Input: part model. Units: mm. Frame: model coordinates. A direction names the side the tool comes from. Coordinates: 2 decimals unless noted, no trailing zeros. Order: outer loops, then holes, each group sorted by start corner. A loop starts at its lowest first (then second) coordinate and runs counter-clockwise, first axis right, second up. Notation, with made-up numbers: M 61,-9.5 L 107,-9.5 A26 ccw 107,12.5 Z; hole C -19.5,46.25 d8. An arc over 180 degrees is marked long. Answer in a Markdown table with one row per item.
Autodesk Inventor part; units mm, degrees
ref_plane "Start plane" through (0, 0, -55) normal (0, 0, 1) x (1, 0, 0)
ref_plane "End plane" through (0, 0, 1555) normal (0, 0, 1) x (1, 0, 0)
ref_plane "Work Plane4" through (55, 0, 1555) normal (-0.7071, 0, 0.7071) x (0.7071, 0, 0.7071)
ref_plane "Start plane" through (0, 0, -55) normal (0, 0, 1) x (1, 0, 0)
ref_plane "End plane" through (0, 0, 1555) normal (0, 0, 1) x (1, 0, 0)
sketch "Sketch2" plane through (0, 0, 0) normal (0, 0, 1) x (1, 0, 0)
  line L0 (-55, 100.8) -> (-14.95, 100.8)
  line L1 (-55, 110) -> (-55, 100.8)
  line L2 (55, 110) -> (-55, 110)
  line L3 (55, 100.8) -> (55, 110)
  line L4 (14.95, 100.8) -> (55, 100.8)
  line L5 (2.95, -88.8) -> (2.95, 88.8)
  line L6 (55, -100.8) -> (14.95, -100.8)
  line L7 (55, -110) -> (55, -100.8)
  line L8 (-55, -100.8) -> (-55, -110)
  line L9 (-14.95, -100.8) -> (-55, -100.8)
  line L10 (-2.95, 88.8) -> (-2.95, -88.8)
  line L11 (0, -154) -> (0, 154) construction
  line L12 (-2.95, -100.8) -> (2.95, -100.8) construction
  arc A0 (-14.95, -100.8) -> (-2.95, -88.8) centre (-14.95, -88.8) ccw
  arc A1 (-2.95, 88.8) -> (-14.95, 100.8) centre (-14.95, 88.8) ccw
  arc A2 (14.95, 100.8) -> (2.95, 88.8) centre (14.95, 88.8) ccw
  arc A3 (2.95, -88.8) -> (14.95, -100.8) centre (14.95, -88.8) ccw
  line L13 (-77, 0) -> (77, 0) construction
  line L14 (-55, -110) -> (55, -110)
  point P0 (-2.95, 100.8)
  point P1 (2.95, 100.8)
  point P2 (0, 0)
  point P3 (0, -100.8)
  point P4 (0, 0)
  dimension "d1" = 220
  dimension "d3" = 9.2
  dimension "d5" = 5.9
  dimension "d7" = 110
  dimension "d13" = 12
  dimension "d14" = 110
  dimension "d15" = 55
extrude "Body" add sketch "Sketch2" along normal up to surface (1610 mm away) from surface at -55
sketch "Sketch3" plane through (0, 0, 0) normal (0, 0, 1) x (1, 0, 0)
  line L0 (0, 0) -> (10, 0)
ref_plane "Work Plane3" through (0, 0, 0) normal (0, -1, 0) x (1, 0, 0)
ref_plane "Work Plane4" through (55, 0, 1555) normal (-0.7071, 0, 0.7071) x (0.7071, 0, 0.7071)
split "Split1" plane through (55, 0, 1555) removes the side toward (-0.7071, 0, 0.7071)
ref_plane "Work Plane5" through (55, 0, -55) normal (-0.7071, 0, -0.7071) x (-0.7071, 0, 0.7071)
split "Split2" plane through (55, 0, -55) removes the side toward (-0.7071, 0, -0.7071)
sketch "Sketch4" plane through (0, 0, 0) normal (0, -1, 0) x (1, 0, 0)
  line L0 (-2, -55) -> (12, -55)
  line L1 (-2, 1555) -> (12, 1555)
  dimension "d19" = 1610
equation "\"d1\" = ParH"
equation "\"d3\" = t2"
equation "\"d7\" = b"
equation "\"d13\" = R1"
equation "\"d14\" = 0.5 * d1"
equation "\"d15\" = 0.5 * d7"
equation "\"d8\" = G_L"
equation "\"b\" = 110"
equation "\"ParH\" = 220"
equation "\"R1\" = 12"
equation "\"G_L\" = d19"
equation "\"t1\" = 5.9"
equation "\"t2\" = 9.2"
equation "\"G_OFFSET_START\" = 55"
equation "\"G_OFFSET_END\" = 55"
equation "\"d16\" = -G_OFFSET_START"
equation "\"d17\" = G_OFFSET_END + B_L"
properties part number "DIN 1025 - IPE 220-1610" material "Steel, Mild"
1) Reachability of faces 4 (the face through (-2.95, 1, 740)), 5 (the face through (35, -100.8, 739)), 6 (the face through (0, 1, 0)) from +Z, -Z, +X, -X, +Y, -Y: full face, straight path, thin tool, end or side. Return the list, or none.
Resolved:
| item | result |
|---|---|
| face 4 | +Z, -Z, -X |
| face 5 | +Z, -Z, +X |
| face 6 | -Z, -X, +Y, -Y |
2) Cut plane A-A, the plane x = 40. Output: boundary loops of the cut face in (y, z), and give its area (3 significant figures).
Resolved:
| item | result |
|---|---|
| outline | M -110,-40 L -100.8,-40 L -100.8,1540 L -110,1540 Z; M 100.8,-40 L 110,-40 L 110,1540 L 100.8,1540 Z |
| area | 29,100 mm2 |
3) Cut plane B-B, the plane z = 1299. Output: boundary loops of the cut face in (x, y).
Resolved:
| item | result |
|---|---|
| outline | M -55,-110 L 55,-110 L 55,-100.8 L 14.95,-100.8 A12 cw 2.95,-88.8 L 2.95,88.8 A12 cw 14.95,100.8 L 55,100.8 L 55,110 L -55,110 L -55,100.8 L -14.95,100.8 A12 cw -2.95,88.8 L -2.95,-88.8 A12 cw -14.95,-100.8 L -55,-100.8 Z |
4) Cut plane C-C, the plane y = 56.5. Output: boundary loops of the cut face in (x, z).
Resolved:
| item | result |
|---|---|
| outline | M -2.95,2.95 L 2.95,-2.95 L 2.95,1502.95 L -2.95,1497.05 Z |
5) Contact query for flat-ended pins moving along their axis: pin 1 (4 mm diameter, centred on y = 55.5, z = 863, fed in from +X); pin 2 (2 mm diameter, centred on y = 23.5, z = 164, fed in from -X). Output: stop coordinate, or through.
Resolved:
| item | result |
|---|---|
| pin 1 | stops at x = 2.95 |
| pin 2 | stops at x = -2.95 |
6) Material intervals for probe 1 along Y at (x, z) = (-43, 163); probe 2 along Y at (x, z) = (-13, 580.5); probe 3 along X at (y, z) = (79.5, 497.5), sorted ascending.
Resolved:
| item | result |
|---|---|
| probe 1 | y = -110 to -100.8, 100.8 to 110 |
| probe 2 | y = -110 to -100.64, 100.64 to 110 |
| probe 3 | x = -2.95 to 2.95 |
7) Mould query, pull axis Y, two halves, no side actions, for faces 1 (the face through (1, 110, 739)), 2 (the face through (-35, 100.8, 740)), 3 (the face through (0, -1, 1500)). Classes: +Y half, -Y half, draft (parallel to the pull), parting line (faces both ways), or undercut.
Resolved:
| item | result |
|---|---|
| face 1 | +Y half |
| face 2 | undercut |
| face 3 | draft |
